Input: dimensioned drawing with shaded views. Units: mm. Origin: part minimum x, y, z. Coordinates: 2 decimals unless noted, no trailing zeros. Order: outer loops, then holes, each group sorted by start corner. A loop starts at its lowest first (then second) coordinate and runs counter-clockwise, first axis right, second up.
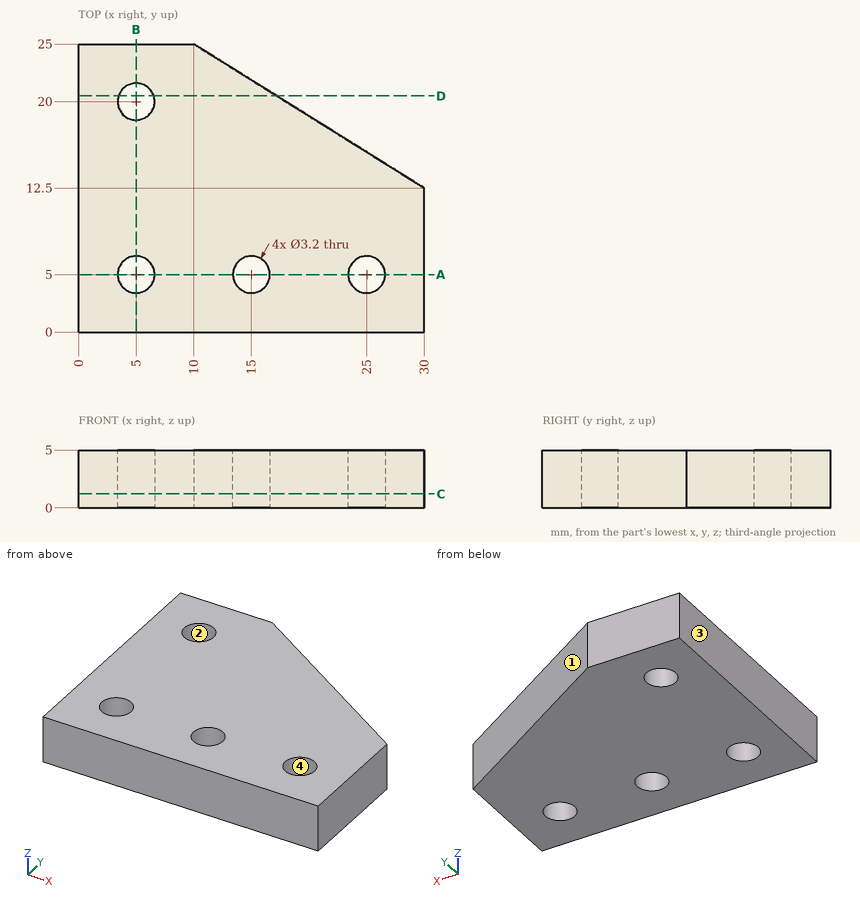
1. Section query A-A on y = 5. Return loops of the section in (x, z).
Findings:
outline: (0, 0) - (3.4, 0) - (3.4, 5) - (0, 5) - close; (6.6, 0) - (13.4, 0) - (13.4, 5) - (6.6, 5) - close; (16.6, 0) - (23.4, 0) - (23.4, 5) - (16.6, 5) - close; (26.6, 0) - (30, 0) - (30, 5) - (26.6, 5) - close
2. Draft query along Y for the marked faces 1, 2, 3 and 4. Return one class per face: released by +Y, released by -Y, zero draft, split by the parting line, or undercut.
Findings:
face 1: released by +Y
face 2: undercut
face 3: zero draft
face 4: undercut
3. Ray query, line 1 (Y direction, x = 5, z = 3.05); line 2 (X direction, y = 4, z = 2.25); line 3 (Y direction, x = 6, z = 0.2). Return the intervals inside material, ascending.
Findings:
line 1: y = 0 to 3.4, 6.6 to 18.4, 21.6 to 25
line 2: x = 0 to 3.75, 6.25 to 13.75, 16.25 to 23.75, 26.25 to 30
line 3: y = 0 to 3.75, 6.25 to 18.75, 21.25 to 25
4. Section query B-B on x = 5. Return loops of the section in (y, z).
Findings:
outline: (0, 0) - (3.4, 0) - (3.4, 5) - (0, 5) - close; (6.6, 0) - (18.4, 0) - (18.4, 5) - (6.6, 5) - close; (21.6, 0) - (25, 0) - (25, 5) - (21.6, 5) - close
5. Section query C-C on z = 1.2. Return loops of the section in (x, y).
Findings:
outline: (0, 0) - (30, 0) - (30, 12.5) - (10, 25) - (0, 25) - close; hole circle Ø3.2 at (5, 5); hole circle Ø3.2 at (5, 20); hole circle Ø3.2 at (15, 5); hole circle Ø3.2 at (25, 5)
6. Section query D-D on y = 20.5. Return loops of the section in (x, z), plus the area to 3 significant figures.
Findings:
outline: (0, 0) - (3.48, 0) - (3.48, 5) - (0, 5) - close; (6.52, 0) - (17.2, 0) - (17.2, 5) - (6.52, 5) - close
area: 70.8 mm2
